Input: part model. Units: mm. Frame: model coordinates. A direction names the side the tool comes from. Coordinates: 2 decimals unless noted, no trailing zeros. Write each loop counter-clockwise with the first axis right and the second up, starting at its lowest first coordinate (ties: lowest second). Pieces come first, ordered by that corner, then holes. Notation, with made-up numbers: M -2.5,-17.5 L 6.5,-17.5 A36 cw 6.5,16.5 Z; hole C -18,57 d8. An arc over 180 degrees is marked long. Use one line per item in the form item = value.
from build123d import *

# Parameters (mm, degrees)
CROQUIS2_W                                           = 47.2
CROQUIS2_H                                           = 18
SALIENTE_EXTRUIR1_DEPTH                              = 12
SALIENTE_EXTRUIR2_DEPTH                              = 5
SALIENTE_EXTRUIR2_DEPTH_BACK                         = 5
REFRENTADO_PARA_TORNILLO_CON_CABEZA_TRON_D           = 3.2
REFRENTADO_PARA_TORNILLO_CON_CABEZA_TRON_DEPTH       = 30
REFRENTADO_PARA_TORNILLO_CON_CABEZA_TRON_CBORE_D     = 5
REFRENTADO_PARA_TORNILLO_CON_CABEZA_TRON_CBORE_DEPTH = 2.4
REFRENTADO_PARA_TORNILLO_CON_CABEZA_TRON_TIP         = 0.96137699
TALADRO_DE_MARGEN_PARA_M21_D                         = 2
TALADRO_DE_MARGEN_PARA_M21_DEPTH                     = 15
TALADRO_DE_MARGEN_PARA_M21_TIP                       = 0.600860619
CROQUIS14_R                                          = 10
CORTAR_EXTRUIR1_DEPTH                                = 16
REDONDEO1_R                                          = 6
CORTAR_EXTRUIR2_DEPTH                                = 16
REDONDEO2_R                                          = 5
REDONDEO3_R                                          = 5


with BuildPart() as part:
    # Croquis2 → Saliente-Extruir1 (new body)
    with BuildSketch(Plane(origin=(0, 0, 0), x_dir=(1, 0, 0), z_dir=(0, 1, 0))):
        with Locations((17, 0)):
            Rectangle(CROQUIS2_W, CROQUIS2_H)
    extrude(amount=SALIENTE_EXTRUIR1_DEPTH)

    # Croquis4 → Saliente-Extruir2 (add, two sides: drawn at the far end of the back side and taken through both)
    with BuildSketch(Plane(origin=(0, 0, 0), x_dir=(-1, 0, 0), z_dir=(0, 0, -1)).offset(-SALIENTE_EXTRUIR2_DEPTH_BACK)):
        with BuildLine():
            Line((-25.5, 22), (-29.5, 22))
            Line((-29.5, 22), (-29.5, 12))
            Line((-29.5, 12), (-4.5, 12))
            Line((-4.5, 12), (-4.5, 22))
            Line((-4.5, 22), (-8.5, 22))
            ThreePointArc((-8.5, 22), (-17, 13.5), (-25.5, 22))
        make_face()
    extrude(amount=SALIENTE_EXTRUIR2_DEPTH + SALIENTE_EXTRUIR2_DEPTH_BACK)

    # Refrentado para tornillo con cabeza troncocónica de M31
    with Locations(Plane.ZX.offset(12)):
        with Locations((0, 0), (0, 34)):
            CounterBoreHole(REFRENTADO_PARA_TORNILLO_CON_CABEZA_TRON_D / 2, REFRENTADO_PARA_TORNILLO_CON_CABEZA_TRON_CBORE_D / 2, REFRENTADO_PARA_TORNILLO_CON_CABEZA_TRON_CBORE_DEPTH, depth=REFRENTADO_PARA_TORNILLO_CON_CABEZA_TRON_DEPTH)
            with Locations((0, 0, -(REFRENTADO_PARA_TORNILLO_CON_CABEZA_TRON_DEPTH + REFRENTADO_PARA_TORNILLO_CON_CABEZA_TRON_TIP / 2))):  # 118° drill point
                Cone(0, REFRENTADO_PARA_TORNILLO_CON_CABEZA_TRON_D / 2, REFRENTADO_PARA_TORNILLO_CON_CABEZA_TRON_TIP, mode=Mode.SUBTRACT)

    # Taladro de margen para M21
    with Locations(Plane(origin=(6, 22, -3), x_dir=(0, 0, 1), z_dir=(0, 1, 0))):
        with Locations((0, 0), (6, 0), (0, 22), (6, 22)):
            Hole(TALADRO_DE_MARGEN_PARA_M21_D / 2, depth=TALADRO_DE_MARGEN_PARA_M21_DEPTH)
            with Locations((0, 0, -(TALADRO_DE_MARGEN_PARA_M21_DEPTH + TALADRO_DE_MARGEN_PARA_M21_TIP / 2))):  # 118° drill point
                Cone(0, TALADRO_DE_MARGEN_PARA_M21_D / 2, TALADRO_DE_MARGEN_PARA_M21_TIP, mode=Mode.SUBTRACT)

    # Croquis14 → Cortar-Extruir1 (cut)
    with BuildSketch(Plane(origin=(0, 12, 0), x_dir=(1, 0, 0), z_dir=(0, 1, 0))):
        with Locations((43.936945617, 11.477309168)):
            Circle(CROQUIS14_R)
        with Locations((-9.936945617, 11.477309168)):
            Circle(CROQUIS14_R)
        with Locations((43.936945617, -11.477309168)):
            Circle(CROQUIS14_R)
        with Locations((-9.936945617, -11.477309168)):
            Circle(CROQUIS14_R)
    extrude(amount=-CORTAR_EXTRUIR1_DEPTH, mode=Mode.SUBTRACT)

    # Redondeo1
    # the kernel refuses this fillet: 6 mm, written as the material it takes off along each edge
    with BuildSketch(Plane(origin=(-6.6, -8.915795606, -2.050496666), x_dir=(0, 0, 1), z_dir=(0, 1, 0))) as redondeo1_piece_1:
        with BuildLine():
            CenterArc((3.566318242, 6), REDONDEO1_R, 215.701262203, 54.298737797)
            ThreePointArc((-1.306105787, 2.498645393), (-0.564551793, 1.295584483), (0, 0))
            Line((0, 0), (3.566318242, 0))
        make_face()
    extrude(amount=29.831591212, mode=Mode.SUBTRACT)
    with BuildSketch(Plane(origin=(-6.6, -8.915795606, 2.050496666), x_dir=(0, 0, -1), z_dir=(0, 1, 0)), Plane(origin=(40.6, -8.915795606, -2.050496666), x_dir=(0, 0, 1), z_dir=(0, 1, 0))) as redondeo1_piece_2:
        with BuildLine():
            CenterArc((3.566318242, -6), REDONDEO1_R, 90, 54.298737797)
            ThreePointArc((-1.306105787, -2.498645393), (-0.564551793, -1.295584483), (0, 0))
            Line((0, 0), (3.566318242, 0))
        make_face()
    extrude(amount=29.831591212, mode=Mode.SUBTRACT)
    with BuildSketch(Plane(origin=(40.6, -8.915795606, 2.050496666), x_dir=(-0.886226070867775, 0, 0.46325301004339436), z_dir=(0, 1, 0))) as redondeo1_piece_3:
        with BuildLine():
            CenterArc((3.665248765, -5.940082264), REDONDEO1_R, 98.104043871, 54.298737797)
            Line((-1.652107661, -3.160564203), (0, 0))
            ThreePointArc((0, 0), (1.409711063, -0.099862894), (2.819422127, 0))
        make_face()
    extrude(amount=29.831591212, mode=Mode.SUBTRACT)

    # Croquis15 → Cortar-Extruir2 (cut)
    with BuildSketch(Plane(origin=(0, 12, 0), x_dir=(1, 0, 0), z_dir=(0, 1, 0))):
        with BuildLine():
            ThreePointArc((-1.535379674, 6.05387025), (-3.319618886, 0), (-1.535379674, -6.05387025))
            ThreePointArc((-1.535379674, -6.05387025), (-2.691742174, -4.584775013), (-4.101354607, -3.356602453))
            ThreePointArc((-4.101354607, -3.356602453), (-5.546762714, -1.879695859), (-6.405366909, 0))
            ThreePointArc((-6.405366909, 0), (-5.546762714, 1.879695859), (-4.101354607, 3.356602453))
            ThreePointArc((-4.101354607, 3.356602453), (-2.691742174, 4.584775013), (-1.535379674, 6.05387025))
        make_face()
        with BuildLine():
            ThreePointArc((38.101354607, 3.356602453), (36.691742174, 4.584775013), (35.535379674, 6.05387025))
            ThreePointArc((35.535379674, 6.05387025), (37.319618886, 0), (35.535379674, -6.05387025))
            ThreePointArc((35.535379674, -6.05387025), (36.691742174, -4.584775013), (38.101354607, -3.356602453))
            ThreePointArc((38.101354607, -3.356602453), (39.546762714, -1.879695859), (40.405366909, 0))
            ThreePointArc((40.405366909, 0), (39.546762714, 1.879695859), (38.101354607, 3.356602453))
        make_face()
    extrude(amount=-CORTAR_EXTRUIR2_DEPTH, mode=Mode.SUBTRACT)

    # Redondeo2
    redondeo2_edges = [part.edges().sort_by_distance(p)[0] for p in [
        (34.248656848, 6, -9),
        (-0.248656848, 6, -9),
    ]]
    fillet(redondeo2_edges, radius=REDONDEO2_R)

    # Redondeo3
    redondeo3_edges = [part.edges().sort_by_distance(p)[0] for p in [
        (34.248656848, 6, 9),
        (-0.248656848, 6, 9),
    ]]
    fillet(redondeo3_edges, radius=REDONDEO3_R)


solid = part.part
(1) Pull-direction query (X, two-part tool) for faces 1 (the flat face through (4.5, 17, 0)), 2 (the cylindrical face through (33.405, 6.084, 8.346)), 3 (the cylindrical face through (36.11, 10.82, 1.34)); classes: pulls with the +X half, pulls with the -X half, needs draft (parallel to the pull), parting line crosses it, or undercut.
Computed:
face_1 = pulls with the -X half
face_2 = pulls with the +X half
face_3 = undercut
(2) Set-up query: faces 4 (the cylindrical face through (-3.32, 6.08, -0.09)), 5 (the cylindrical face through (7, 14, -3)), 6 (the flat face through (20, 13.7, 5)), 7 (the flat face through (29.5, 17, 0)), 8 (the flat face through (6, 22, 0)). Return all of +Z, -Z, +X, -X, +Y, -Y with unobstructed straight access to the full face (end or side cutting, diameter ignored); none if empty.
Computed:
face_4 = -X, +Y, -Y
face_5 = +Y
face_6 = +Z, +X, -X, +Y
face_7 = +Z, -Z, +X, +Y
face_8 = +Z, -Z, +X, -X, +Y
(3) Section query A-A on y = 6. Return the cut outline in (x, z).
Computed:
outline = M -1.54,-6.05 A10 cw -1.27,-6.49 A5 ccw 3.07,-9 L 30.93,-9 A5 ccw 35.27,-6.49 A10 cw 35.54,-6.05 A11.16 ccw 35.54,6.05 A10 cw 35.27,6.49 A5 ccw 30.93,9 L 3.07,9 A5 ccw -1.27,6.49 A10 cw -1.54,6.05 A11.16 ccw Z; hole C 0,0 d3.2; hole C 34,0 d3.2
(4) Line query: probe 1 along X at (y, z) = (2.75, 0); probe 2 along X at (y, z) = (10.7, 0); probe 3 along Z at (x, y) = (6, 10.25). Output: solid intervals per line, ascending.
Computed:
probe_1 = -3.32 to -1.6, 1.6 to 32.4, 35.6 to 37.32
probe_2 = -3.32 to -2.5, 2.5 to 31.5, 36.5 to 37.32
probe_3 = -9 to -4, -2 to 2, 4 to 9
(5) Section query B-B on x = 0. Return the cut outline in (y, z).
Computed:
outline = M 0,-7.95 L 12,-7.95 L 12,-2.5 L 9.6,-2.5 L 9.6,-1.6 L 0,-1.6 Z; M 0,1.6 L 9.6,1.6 L 9.6,2.5 L 12,2.5 L 12,7.95 L 0,7.95 Z
(6) First-contact query: pin 1 Ø11 at (x, y) = (19.5, 19) entering from -Z; pin 2 Ø2.5 at (x, z) = (33, 1) entering from +Y; pin 3 Ø3 at (x, z) = (0, 0) entering from -Y; pin 4 Ø5 at (y, z) = (18, -0.5) entering from -X. Flat tips, straight axial feed; report the tip coordinate or a pass-through.
Computed:
pin_1 = -5
pin_2 = 12
pin_3 = through
pin_4 = 4.5
(7) Section query C-C on y = 16. Return the cut outline in (x, z), plus the area to 3 significant figures.
Computed:
outline = M 4.5,-5 L 10.98,-5 L 10.98,5 L 4.5,5 Z; M 23.02,-5 L 29.5,-5 L 29.5,5 L 23.02,5 Z; hole C 6,-3 d2; hole C 6,3 d2; hole C 28,-3 d2; hole C 28,3 d2
area = 117 mm^2
(8) Section query D-D on z = -7. Return the cut outline in (x, y), plus the area to 3 significant figures.
Computed:
outline = M -0.93,0 L 34.93,0 L 34.93,12 L -0.93,12 Z
area = 430 mm^2
